Check sheet for the modelled part. Datum: model origin and axes. Units: mm. A direction names the side the tool comes from. Give positions to 0.01 mm unless a question says otherwise; leave off trailing zeros. Loops run counter-clockwise (first coordinate to the right, second up) from the corner with the lowest first, then second, coordinate; pieces in that order, holes last. Notation, with made-up numbers: (-38, -26) -> (-29, -26) arc R8 ccw to (-29, -17) -> close; hole circle Ø3 at (84.25, -39). An arc over 180 degrees is marked (long way). Write each question's results on one line, items separated by ' | '. Start each with the question number.
Item 1: Cross-section at A-A on z = 12. Enter the section's corners in (x, y) (3 decimals).
Item 2: Mould release check, pull along Y, two halves, no side actions. Record for faces 1 (the face through (14, 39, -4.5)), 2 (the face through (12.25, 7.22, 19.68)): pulls with the +Y half, pulls with the -Y half, needs draft (parallel to the pull), parting line crosses it, or undercut.
Item 3: Access from +Z, -Z, +X, -X, +Y, -Y to the whole of each face (thin tool, end or side, straight path). Record for faces 3 (the face through (-12.936, -7.886, 23.052)), 4 (the face through (-1, -9, 28.575)), 5 (the face through (11, 0, 27)).
Item 4: Scan lines: line 1 along X through (y, z) = (0, 8.25) (3 decimals); line 2 along Z through (x, y) = (9.5, 30.5) (3 decimals). Record each from-to range of solid material in increasing order.
Item 5: Gauge pin test, flat ends, axial feed: pin 1 Ø0.9 at (x, z) = (-12, 23) entering from +Y; pin 2 Ø3 at (x, z) = (-2, 23.5) entering from -Y; pin 3 Ø1 at (y, z) = (5.5, 6.5) entering from +X. Record the tip position at first contact, or that the pin passes through.
Autodesk Inventor part; units mm, degrees
ref_plane "YZ Plane" through (0, 0, 0) normal (1, 0, 0) x (0, 1, 0)
ref_plane "XZ Plane" through (0, 0, 0) normal (0, 1, 0) x (-1, 0, 0)
ref_plane "XY Plane" through (0, 0, 0) normal (0, 0, 1) x (1, 0, 0)
sketch "Sketch1" plane through (0, 0, 0) normal (0, 0, 1) x (1, 0, 0)
  circle A0 centre (0, 0) radius 41.275
  circle A1 centre (0, 0) radius 47.625
  dimension "d0" = 82.55
  dimension "d1" = 6.35
extrude "Extrusion1" add sketch "Sketch1" along normal blind 25.4
sketch "Sketch2" plane through (0, 0, 25.4) normal (0, 0, 1) x (1, 0, 0)
  circle A0 centre (0, 0) radius 47.625
extrude "Extrusion2" add sketch "Sketch2" along normal blind 3.175
sketch "Sketch3" plane through (0, 0, 25.4) normal (0, 0, -1) x (-1, 0, 0)
  line L0 (11, 6) -> (-11, 6)
  line L1 (-11, 6) -> (-11, -6)
  line L2 (-11, -6) -> (11, -6)
  line L3 (11, -6) -> (11, 6)
  line L4 (11, 6) -> (-11, -6) construction
  line L5 (-11, 6) -> (11, -6) construction
  line L6 (-10.6662, 8.8412) -> (10.6662, 8.8412)
  line L7 (13.8412, 5.6662) -> (13.8412, -5.6662)
  line L8 (10.6662, -8.8412) -> (-10.6662, -8.8412)
  line L9 (-13.8412, -5.6662) -> (-13.8412, 5.6662)
  arc A0 (-10.6662, 8.8412) -> (-13.8412, 5.6662) centre (-10.6662, 5.6662) ccw
  arc A1 (-13.8412, -5.6662) -> (-10.6662, -8.8412) centre (-10.6662, -5.6662) ccw
  arc A2 (10.6662, -8.8412) -> (13.8412, -5.6662) centre (10.6662, -5.6662) ccw
  arc A3 (13.8412, 5.6662) -> (10.6662, 8.8412) centre (10.6662, 5.6662) ccw
  point P0 (0, 0)
  dimension "d6" = 22
  dimension "d7" = 12
  dimension "d8" = 3.175
extrude "Extrusion3" add sketch "Sketch3" along normal blind 6.35
chamfer "Chamfer1" distance 1.5875 angle 45 8 edges at (0, 8.8412, 19.05) (12.9113, 7.9113, 19.05) (13.8412, 0, 19.05) (12.9113, -7.9113, 19.05) (0, -8.8412, 19.05) (-12.9113, -7.9113, 19.05) (-13.8412, 0, 19.05) (-12.9113, 7.9113, 19.05)
sketch "Sketch5" plane through (-13.8412, -5.6662, 25.4) normal (-1, 0, 0) x (0, 0, 1)
  line L0 (-0.1094, 0) -> (-8.0486, 0)
  line L1 (-8.0486, 0) -> (-8.0486, 11.3324)
  line L2 (-8.0486, 11.3324) -> (-0.1094, 11.3324)
  line L3 (-0.1094, 11.3324) -> (-0.1094, 0)
  point P0 (-25.4, 5.6662)
extrude "Extrusion5" cut sketch "Sketch5" against normal blind 28.575
sketch "Sketch6" plane through (0, 0, 0) normal (0, 0, -1) x (-1, 0, 0)
  circle A0 centre (0, 0) radius 47.625
  circle A1 centre (0, 0) radius 41.275
extrude "Extrusion6" add sketch "Sketch6" along normal blind 4.5
chamfer "Chamfer2" distance 1.5875 angle 45 1 edges at (-47.625, 0, 28.575)
fillet "Fillet2" radius 1.5875 1 edges at (-46.0375, 0, 28.575)
fillet "Fillet3" radius 1.5875 1 edges at (-47.625, 0, 26.9875)
sketch "Sketch7" plane through (0, 0, 25.4) normal (0, 0, -1) x (-1, 0, 0)
  circle A0 centre (0, 0) radius 41.275
  line L0 (-10.6662, 8.8412) -> (10.6662, 8.8412)
  arc A1 (13.8412, 5.6662) -> (10.6662, 8.8412) centre (10.6662, 5.6662) ccw
  line L1 (13.8412, 5.6662) -> (13.8412, -5.6662)
  arc A2 (10.6662, -8.8412) -> (13.8412, -5.6662) centre (10.6662, -5.6662) ccw
  line L2 (10.6662, -8.8412) -> (-10.6662, -8.8412)
  arc A3 (-13.8412, -5.6662) -> (-10.6662, -8.8412) centre (-10.6662, -5.6662) ccw
  line L3 (-13.8412, -5.6662) -> (-13.8412, 5.6662)
  arc A4 (-10.6662, 8.8412) -> (-13.8412, 5.6662) centre (-10.6662, 5.6662) ccw
  line L4 (10.6662, 7.2537) -> (10.6662, 8.8412)
  arc A5 (12.2537, 5.6662) -> (10.6662, 7.2537) centre (10.6662, 5.6662) ccw
  line L5 (13.8412, 5.6662) -> (12.2537, 5.6662)
  arc A6 (13.8412, 5.6662) -> (10.6662, 8.8412) centre (10.6662, 5.6662) ccw
  line L6 (-10.6662, 7.2537) -> (10.6662, 7.2537)
  line L7 (-12.2537, 5.6662) -> (-11, 5.6662)
  line L8 (-11, 5.6662) -> (-11, 6)
  line L9 (-11, 6) -> (11, 6)
  line L10 (11, 6) -> (11, 5.6662)
  line L11 (11, 5.6662) -> (12.2537, 5.6662)
  arc A7 (12.2537, 5.6662) -> (10.6662, 7.2537) centre (10.6662, 5.6662) ccw
  line L12 (-10.6662, 7.2537) -> (10.6662, 7.2537)
  arc A8 (-10.6662, 7.2537) -> (-12.2537, 5.6662) centre (-10.6662, 5.6662) ccw
  line L13 (-10.6662, 8.8412) -> (-10.6662, 7.2537)
  line L14 (-10.6662, 7.2537) -> (10.6662, 7.2537)
  line L15 (10.6662, 7.2537) -> (10.6662, 8.8412)
  line L16 (10.6662, 8.8412) -> (-10.6662, 8.8412)
  line L17 (-11, 6) -> (11, 6)
  line L18 (10.6662, 8.8412) -> (-10.6662, 8.8412)
  line L19 (11, 5.6662) -> (12.2537, 5.6662)
  line L20 (10.6662, 8.8412) -> (-10.6662, 8.8412)
  line L21 (-10.6662, -8.8412) -> (10.6662, -8.8412)
  line L22 (10.6662, -8.8412) -> (-10.6662, -8.8412)
  arc A9 (13.8412, 5.6662) -> (10.6662, 8.8412) centre (10.6662, 5.6662) ccw
  arc A10 (13.8412, 5.6662) -> (10.6662, 8.8412) centre (10.6662, 5.6662) ccw
  line L23 (10.6662, -8.8412) -> (10.6662, -7.2537)
  arc A11 (10.6662, -8.8412) -> (13.8412, -5.6662) centre (10.6662, -5.6662) ccw
  arc A12 (-13.8412, -5.6662) -> (-10.6662, -8.8412) centre (-10.6662, -5.6662) ccw
  arc A13 (-10.6662, 8.8412) -> (-13.8412, 5.6662) centre (-10.6662, 5.6662) ccw
  arc A14 (-10.6662, 8.8412) -> (-13.8412, 5.6662) centre (-10.6662, 5.6662) ccw
  line L24 (11, -6) -> (11, 6)
  line L25 (11, 5.6662) -> (11, 6)
  line L26 (11, 6) -> (-11, 6)
  line L27 (-11, 5.6662) -> (-11, -5.6662)
  line L28 (-11, 6) -> (-11, 5.6662)
  line L29 (-11, 5.6662) -> (-13.8412, 5.6662)
  line L30 (-11, -5.6662) -> (-13.8412, -5.6662)
  line L31 (-13.8412, -5.6662) -> (-11, -5.6662)
  line L32 (-11, -6) -> (-11, -5.6662)
  line L33 (-11, -5.6662) -> (-11, -6)
  line L34 (-11, -6) -> (11, -6)
  line L35 (11, -5.6662) -> (11, -6)
  line L36 (11, -6) -> (11, -5.6662)
  line L37 (13.8412, -5.6662) -> (11, -5.6662)
  line L38 (11, -5.6662) -> (13.8412, -5.6662)
  line L39 (10.6662, 7.2537) -> (10.6662, 8.8412)
  arc A15 (13.8412, 5.6662) -> (10.6662, 8.8412) centre (10.6662, 5.6662) ccw
  arc A16 (-10.6662, 8.8412) -> (-13.8412, 5.6662) centre (-10.6662, 5.6662) ccw
  line L40 (10.6662, 8.8412) -> (-10.6662, 8.8412)
  line L41 (11, 6) -> (-11, 6)
  line L42 (-11, 5.6662) -> (-11, 6)
  line L43 (-13.8412, 5.6662) -> (-12.2537, 5.6662)
  line L44 (-11, 5.6662) -> (-13.8412, 5.6662)
  line L45 (13.8412, 5.6662) -> (13.8412, -5.6662)
  line L46 (13.8412, 5.6662) -> (11, 5.6662)
sketch "Sketch8" plane through (0, 0, 28.575) normal (0, 0, 1) x (1, 0, 0)
  line L0 (0, 0) -> (18.6341, 0)
  line L1 (18.6341, 0) -> (18.6341, -16.7894)
  line L2 (18.6341, -16.7894) -> (18.6341, 0)
  line L3 (18.6341, 0) -> (18.6341, 16.7894)
  line L4 (18.6341, 16.7894) -> (24.9841, 16.7894)
  line L5 (24.9841, 16.7894) -> (24.9841, -16.7894)
  line L6 (24.9841, -16.7894) -> (18.6341, -16.7894)
  dimension "d28" = 16.7894
  dimension "d29" = 6.35
  dimension "d30" = 33.5788
extrude "Extrusion7" add sketch "Sketch8" along normal blind 63.5
fillet "Fillet4" radius 3.175 3 edges at (24.9841, 0, 92.075) (21.8091, -16.7894, 92.075) (21.8091, 16.7894, 92.075)
sketch "Sketch10" plane through (0, 0, 25.4) normal (0, 0, -1) x (-1, 0, 0)
  line L0 (11, 6) -> (-11, 6)
  line L1 (-11, -6) -> (11, -6)
  line L2 (-11, 6) -> (11, 6)
  line L3 (11, 6) -> (11, -6)
  line L4 (11, -6) -> (-11, -6)
  line L5 (-11, -6) -> (-11, 6)
  point P0 (0, 0)
extrude "Extrusion9" cut sketch "Sketch10" against normal up to surface (3.175 mm away)
sketch "Sketch11" plane through (18.6341, -16.7894, 28.575) normal (-1, 0, 0) x (0, 0, 1)
  line L0 (48.8213, 27.8052) -> (49.1551, 27.8061)
  line L1 (37.2166, 5.7727) -> (37.1859, 16.7726)
  line L2 (49.1551, 27.8061) -> (37.2166, 27.8061)
  line L3 (37.2166, 27.8061) -> (37.2166, 5.7727)
  line L4 (37.2166, 5.7727) -> (49.1551, 5.7727)
  line L5 (49.1551, 5.7727) -> (49.1551, 27.8061)
  point P0 (-28.575, 16.7894)
extrude "Extrusion10" cut sketch "Sketch11" against normal up to surface (6.35 mm away)
sketch "Sketch12" plane through (18.6341, -16.7894, 28.575) normal (-1, 0, 0) x (0, 0, 1)
  line L0 (37.2166, 5.7727) -> (37.2166, 27.8061)
  line L1 (37.2166, 27.8061) -> (49.1551, 27.8061)
  line L2 (49.1551, 27.8061) -> (49.1551, 5.7727)
  line L3 (49.1551, 5.7727) -> (37.2166, 5.7727)
  arc A0 (63.5, 30.4038) -> (60.325, 33.5788) centre (60.325, 30.4038) ccw
  line L4 (0, 33.5788) -> (60.325, 33.5788)
  line L5 (0, 0) -> (0, 33.5788)
  line L6 (0, 0) -> (60.325, 0)
  arc A1 (60.325, 0) -> (63.5, 3.175) centre (60.325, 3.175) ccw
  line L7 (63.5, 30.4038) -> (63.5, 3.175)
  line L8 (37.2166, 27.8061) -> (37.2166, 5.7727)
  line L9 (49.1551, 27.8061) -> (37.2166, 27.8061)
  line L10 (37.2166, 27.8061) -> (37.2166, 5.7727)
  line L11 (37.2166, 5.7727) -> (49.1551, 5.7727)
  line L12 (49.1551, 5.7727) -> (49.1551, 27.8061)
  point P0 (-28.575, 16.7894)
sketch "Sketch13" plane through (0, 0, 92.075) normal (0, 0, 1) x (1, 0, 0)
  circle A0 centre (0, 0) radius 41.275
  line L0 (34.9461, 21.9635) -> (13.1232, 21.9635)
  line L1 (13.1232, 21.9635) -> (13.1232, -23.4108)
  line L2 (13.1232, -23.4108) -> (34.9461, -23.4108)
  line L3 (34.9461, -23.4108) -> (34.9461, 21.9635)
  point P0 (33.9936, -23.4108)
  point P1 (34.9461, -21.9635)
extrude "Extrusion11" cut sketch "Sketch13" against normal up to surface (63.5 mm away) contours L3 A0 L2 L1 L0
properties part number "Base"
Answer sheet:
1) outline: circle Ø95.25 at (0, 0); hole circle Ø82.55 at (0, 0)
2) face 1: needs draft | face 2: undercut
3) face 3: -Z | face 4: +Z, +X, -X, +Y, -Y | face 5: +Z, -Z
4) line 1: x = -47.625 to -41.275, 41.275 to 47.625 | line 2: z = 25.4 to 28.575
5) pin 1: stops at y = 46.2 | pin 2: stops at y = -47.62 | pin 3: stops at x = 47.36
